```python
from build123d import *


with BuildPart() as part:
    # Sketch1 → Revolve2 (revolve)
    with BuildSketch(Plane.XY):
        with BuildLine():
            Line((-21.346613546, 51.322709163), (-31, 0))
            Line((-31, 0), (-13, 0))
            Line((-13, 0), (-13, 38))
            Line((-13, 38), (0, 38))
            Line((0, 38), (0, 62.22310757))
            add(Edge.make_bspline(
                [(-21.346613546, 51.322709163), (-12.732751992, 60.593465444), (0, 62.22310757)],
                knots=[0, 0, 0, 1, 1, 1], degree=2))
        make_face()
    revolve(axis=Axis((0, 62.22310757, 0), (0, -1, 0)))

    # Sketch3 → Revolve3 (revolve)
    with BuildSketch(Plane.XY):
        with BuildLine():
            Line((-19.124549702, 38.552742214), (-75.621657411, 67.624527958))
            Line((-75.621657411, 67.624527958), (-72.008511604, 74.646191148))
            add(Edge.make_bspline(
                [(-72.008511604, 74.646191148), (-46.325833762, 68.784299288), (-26.392991631, 51.173757302)],
                knots=[0, 0, 0, 1, 1, 1], degree=2))
            Line((-26.392991631, 51.173757302), (-15.511403895, 45.574405405))
            Line((-15.511403895, 45.574405405), (-19.124549702, 38.552742214))
        make_face()
    revolve(axis=Axis((-19.124549702, 38.552742214, 0), (-0.889184528, 0.457548769, 0)))


solid = part.part
```
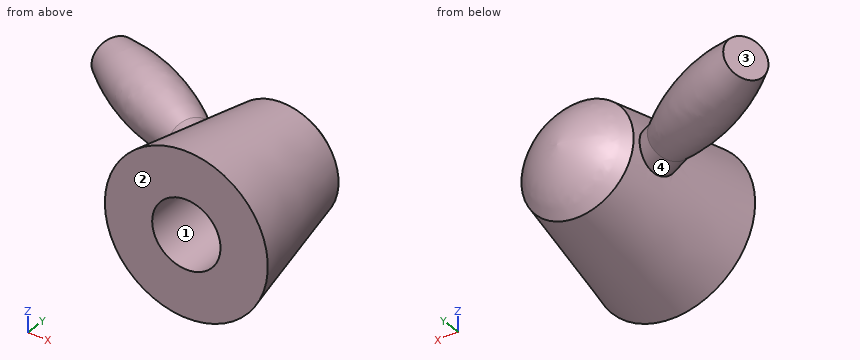
Geometry check sheet. Reference: the model listing, model coordinates, mm. Face numbers are marked on the shaded views. Coordinates: 2 decimals unless noted, no trailing zeros. Order: outer loops, then holes, each group sorted by start corner. A loop starts at its lowest first (then second) coordinate and runs counter-clockwise, first axis right, second up. Notation, with made-up numbers: M 84.25,36 L 111.25,36 A37 cw 111.25,72 Z; hole C 4,-22 d8. An arc over 180 degrees is marked long. One line per question, with ' | ' between items. Start each with the question number.
Item 1: Draft check along Y on the marked faces 1, 2, 3 and 4. Enter one of: pulls with the +Y half, pulls with the -Y half, needs draft (parallel to the pull), parting line crosses it, or undercut.
Item 2: Material ranges on L1, parallel to X at y = 12, z = 0; L2, parallel to Z at x = 0, y = 22; L3, parallel to X at y = 55.5, z = -0.5, recorded low to high. Write a range as [from, to].
Item 3: Cross-section at A-A on y = 22. Enter the section's corners in (x, z), then the cut area to 3 significant figures.
Item 4: Cross-section at B-B on y = 14. Enter the section's corners in (x, z).
Item 5: Gauge pin test, flat ends, axial feed: pin 1 (1.5 mm diameter, centred on x = -3.5, z = 6, fed in from -Y); pin 2 (1 mm diameter, centred on x = -8, y = 32, fed in from +Z); pin 3 (5 mm diameter, centred on y = 37, z = -10.5, fed in from -X). Record the tip position at first contact, or that the pin passes through.
Findings:
1) face 1: needs draft | face 2: pulls with the -Y half | face 3: pulls with the +Y half | face 4: undercut
2) L1: x = [-28.74, -13], [13, 28.74] | L2: z = [-26.86, -13], [13, 26.86] | L3: x = [-73.01, -31.62], [-16.75, 16.75]
3) outline: C 0,0 d53.72; hole C 0,0 d26 | area: 1,740 mm²
4) outline: C 0,0 d56.73; hole C 0,0 d26
5) pin 1: stops at y = 38 | pin 2: stops at z = 23.86 | pin 3: stops at x = -22.8
